```python
from build123d import *

# Parameters (mm, degrees)
F1_DEPTH = 3
F2_R     = 2.99999


# Not quite as in the source:
# - a fillet or chamfer is up to 0.001 mm smaller than in the source, because OpenCascade refuses the exact size


with BuildPart() as f1:
    # F0 (on Front) → F1 (new body, symmetric)
    with BuildSketch(Plane.XZ):
        Polygon((50, 0), (0, 0), (6.0951397114, -19.0486028857), (50, -5), align=None)
    extrude(amount=F1_DEPTH, both=True)

    # F2 (radius 3 in the source; OpenCascade refuses exactly that, so slightly less here)
    f2_edges = [f1.edges().sort_by_distance(p)[0] for p in [
        (28.04757, -3, -12.024301),
        (28.04757, 3, -12.024301),
    ]]
    fillet(f2_edges, radius=F2_R)


solid = f1.part
```
Read the model definition and answer for the solid it produces. Units are mm, in the model's axes. Coordinates: 2 decimals unless noted, no trailing zeros. Loops run counter-clockwise (first coordinate to the right, second up) from the corner with the lowest first, then second, coordinate; pieces in that order, holes last. Notation, with made-up numbers: (-31.5, 59) - (-7.5, 59) arc R9 cw to (-7.5, 65) - close; hole circle Ø5 at (0, -7). An arc over 180 degrees is marked (long way). Answer in a Markdown table with one row per item.
1. Find section A-A, the plane y = 2.25. Write down the section's boundary in (x, z), then the cut area to 3 significant figures.
Conclusion:
| item | result |
|---|---|
| outline | (0, 0) - (5.79, -18.08) - (50, -3.93) - (50, 0) - close |
| area | 539 mm² |
2. Find section B-B, the plane y = -0.5. Write down the section's boundary in (x, z).
Conclusion:
| item | result |
|---|---|
| outline | (0, 0) - (6.08, -19.01) - (50, -4.96) - (50, 0) - close |
3. Straight lines are drawn through the part: line 1 (Z direction, x = 15, y = 0.25); line 2 (Z direction, x = 44.5, y = 1); line 3 (Y direction, x = 8, z = -16). For each, find the intervals that lie inside material, in ascending order.
Conclusion:
| item | result |
|---|---|
| line 1 | z = -16.19 to 0 |
| line 2 | z = -6.58 to 0 |
| line 3 | y = -2.92 to 2.92 |
